Input: part model. Units: mm. Frame: model coordinates. A direction names the side the tool comes from. Coordinates: 2 decimals unless noted, no trailing zeros. Order: outer loops, then holes, each group sorted by start corner. A loop starts at its lowest first (then second) coordinate and runs counter-clockwise, first axis right, second up.
from build123d import *

# Parameters (mm, degrees)
ESQUISSE1_R             = 45
EXTRUSION1_DEPTH        = 3
ESQUISSE2_R             = 6.75
ESQUISSE2_R_2           = 3.75
ESQUISSE2_R_3           = 5
EXTRUSION2_DEPTH        = 4
ESQUISSE3_R             = 2.1
ENL_V_MAT_EXTRU_1_DEPTH = 8


with BuildPart() as part:
    # Esquisse1 → Extrusion1 (new body)
    with BuildSketch(Plane(origin=(0, 0, 0), x_dir=(1, 0, 0), z_dir=(0, 1, 0))):
        Circle(ESQUISSE1_R)
    extrude(amount=-EXTRUSION1_DEPTH)

    # Esquisse2 → Extrusion2 (add)
    with BuildSketch(Plane.XZ.offset(3)):
        Circle(ESQUISSE2_R)
        Circle(ESQUISSE2_R_2, mode=Mode.SUBTRACT)
        with Locations((-35, 0)):
            Circle(ESQUISSE2_R_3)
        with Locations((17.5, 30.310889132)):
            Circle(ESQUISSE2_R_3)
        with Locations((17.5, -30.310889132)):
            Circle(ESQUISSE2_R_3)
    extrude(amount=EXTRUSION2_DEPTH)

    # Esquisse3 → Enlèv. mat.-Extru.1 (cut, through all)
    with BuildSketch(Plane(origin=(0, 0, 0), x_dir=(1, 0, 0), z_dir=(0, 1, 0))):
        Circle(ESQUISSE3_R)
    extrude(amount=-ENL_V_MAT_EXTRU_1_DEPTH, mode=Mode.SUBTRACT)


solid = part.part
Item 1: Cut plane D-D on x = 17.5. Return loops of the section in (y, z).
Response values:
outline: (-7, -35.31) - (-3, -35.31) - (-3, -41.46) - (0, -41.46) - (0, 41.46) - (-3, 41.46) - (-3, 35.31) - (-7, 35.31) - (-7, 25.31) - (-3, 25.31) - (-3, -25.31) - (-7, -25.31) - close
Item 2: Pin query (flat end, axial travel): pin 1 Ø7 at (x, z) = (0, 0) entering from -Y; pin 2 Ø1 at (x, y) = (16.5, -3) entering from +Z. Return the tip coordinate at first contact, or that it passes through.
Response values:
pin 1: stops at y = -3
pin 2: stops at z = 42.06
Item 3: Ray query, probe 1 along Z at (x, y) = (0, -1.2); probe 2 along Y at (x, z) = (27, 16). Return the intervals inside material, ascending.
Response values:
probe 1: z = -45 to -2.1, 2.1 to 45
probe 2: y = -3 to 0
Item 4: Access query for faces 1 (the face through (2.003, -1.479, -0.631)), 2 (the face through (-1.46, -4.97, -6.59)). Directions: +Z, -Z, +X, -X, +Y, -Y. A direction counts if a zero-diameter tool reaches every point of the face in a straight line with its end or side. Return the directions, or none.
Response values:
face 1: +Y, -Y
face 2: -Y
Item 5: Cut plane B-B on x = 0. Return loops of the section in (y, z).
Response values:
outline: (-7, -6.75) - (-3, -6.75) - (-3, -45) - (0, -45) - (0, -2.1) - (-3, -2.1) - (-3, -3.75) - (-7, -3.75) - close; (-7, 3.75) - (-3, 3.75) - (-3, 2.1) - (0, 2.1) - (0, 45) - (-3, 45) - (-3, 6.75) - (-7, 6.75) - close
Item 6: Cut plane A-A on z = 0. Return loops of the section in (x, y), then the cut area to 3 significant figures.
Response values:
outline: (-45, -3) - (-40, -3) - (-40, -7) - (-30, -7) - (-30, -3) - (-6.75, -3) - (-6.75, -7) - (-3.75, -7) - (-3.75, -3) - (-2.1, -3) - (-2.1, 0) - (-45, 0) - close; (2.1, -3) - (3.75, -3) - (3.75, -7) - (6.75, -7) - (6.75, -3) - (45, -3) - (45, 0) - (2.1, 0) - close
area: 321 mm2
Item 7: Cut plane C-C on y = -1.25. Return loops of the section in (x, z), then the cut area to 3 significant figures.
Response values:
outline: circle Ø90 at (0, 0); hole circle Ø4.2 at (0, 0)
area: 6,350 mm2
Item 8: Draft query along Z for faces 3 (the face through (20.188, -4.972, 34.527)), 4 (the face through (-35, -7, 0)), 5 (the face through (-40, -5, 0)). Return one class per face: pulls with the +Z half, pulls with the -Z half, needs draft (parallel to the pull), parting line crosses it, or undercut.
Response values:
face 3: undercut
face 4: needs draft
face 5: parting line crosses it
